Build history of the part. All positions in model axes, mm. Face numbers are marked on the shaded views. A direction names the side the tool comes from. Round coordinates to 2 decimals unless told otherwise and drop trailing zeros. Order: outer loops, then holes, each group sorted by start corner. A loop starts at its lowest first (then second) coordinate and runs counter-clockwise, first axis right, second up. Notation, with made-up numbers: (-38, -7.75) -> (-24, -7.75) arc R6 ccw to (-24, -0.75) -> close; hole circle Ø3 at (73.25, -21.75). An arc over 180 degrees is marked (long way). Use a Markdown table: item, result. Add a question column.
Item 1: Two-plate mould, pull along Z, no slides. Class the marked faces 6, 7 and 8: released by +Z, released by -Z, zero draft, split by the parting line, or undercut.
Item 2: Slice it at D-D, the plane y = 19. Give the cut face in (x, z) (3 decimals), plus the area to 3 significant figures.
Item 3: Slice it at A-A, the plane y = 9.2. Give the cut face in (x, z) (3 decimals), plus the area to 3 significant figures.
Item 4: Pin check, flat tips, straight feed: pin 1 (10 mm diameter, centred on x = -38, y = 24, fed in from -Z); pin 2 (1.5 mm diameter, centred on y = 23.5, z = 27, fed in from +X); pin 3 (10 mm diameter, centred on x = -7, y = 26.5, fed in from +Z). Stop position of each tip, or through.
Item 5: Slice it at B-B, the plane z = 3.02. Give the cut face in (x, y).
Item 6: Slice it at C-C, the plane x = -37. Give the cut face in (y, z) (3 decimals), plus the area to 3 significant figures.
Item 7: Probe L1, parallel to Y at x = -12.75, z = 3.02; L2, parallel to Y at x = -34, z = 25 (3 decimals); L3, parallel to Z at x = -17.5, y = 14.5 (3 decimals). List the from-to ranges inside material, lowest first.
Item 8: 3-axis set-ups, long thin cutter, end or side, ignore diameter. For the marked faces 1, 2, 3, 4 and 5: which of +Z, -Z, +X, -X, +Y, -Y reach the whole face in a straight line?
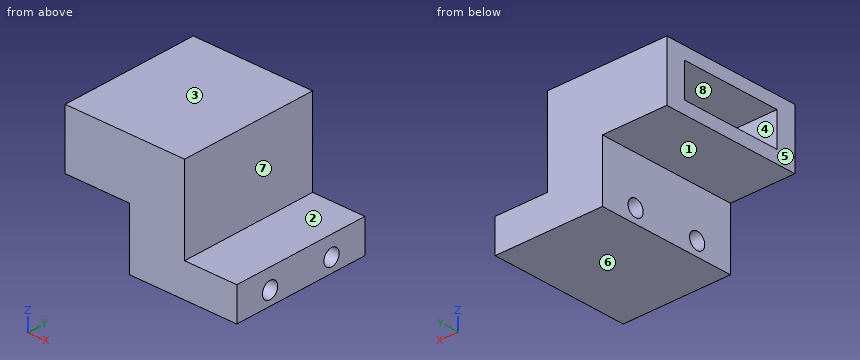
from build123d import *

# Parameters (mm, degrees)
BOSS_EXTRUDE1_DEPTH = 35.4
SKETCH2_W           = 8.63
SKETCH2_H           = 25.55
CUT_EXTRUDE1_DEPTH  = 30
SKETCH3_R           = 2.1
CUT_EXTRUDE2_DEPTH  = 64.958508207


with BuildPart() as part:
    # Sketch1 → Boss-Extrude1 (new body)
    with BuildSketch(Plane(origin=(0, 0, 0), x_dir=(1, 0, 0), z_dir=(0, 1, 0))):
        Polygon((1.0173917, 0.48), (-26.48, 0.48), (-26.48, -15), (-31.48, -15), (-43, -15), (-43, -30), (-12.38, -30), (-12.38, -8.02), (-11.48, -8.02), (1.0173917, -8.02), align=None)
    extrude(amount=BOSS_EXTRUDE1_DEPTH)

    # Sketch2 → Cut-Extrude1 (cut)
    with BuildSketch(Plane.ZY.offset(43)):
        with Locations((22.5, 17.7)):
            Rectangle(SKETCH2_W, SKETCH2_H)
    extrude(amount=-CUT_EXTRUDE1_DEPTH, mode=Mode.SUBTRACT)

    # Sketch3 → Cut-Extrude2 (cut, through all)
    with BuildSketch(Plane(origin=(1.0173917, 0, 0), x_dir=(0, 0, -1), z_dir=(1, 0, 0))):
        with Locations((-3.02, 9.2)):
            Circle(SKETCH3_R)
        with Locations((-3.02, 26.2)):
            Circle(SKETCH3_R)
    extrude(amount=-CUT_EXTRUDE2_DEPTH, mode=Mode.SUBTRACT)


solid = part.part
Check sheet entries:
| question | item | result |
|---|---|---|
| 1 | face 6 | released by -Z |
| 1 | face 7 | zero draft |
| 1 | face 8 | undercut |
| 2 | outline | (-43, 15) -> (-26.48, 15) -> (-26.48, -0.48) -> (1.017, -0.48) -> (1.017, 8.02) -> (-12.38, 8.02) -> (-12.38, 30) -> (-43, 30) -> (-43, 26.815) -> (-13, 26.815) -> (-13, 18.185) -> (-43, 18.185) -> close |
| 2 | area | 533 mm2 |
| 3 | outline | (-43, 15) -> (-26.48, 15) -> (-26.48, 5.12) -> (1.017, 5.12) -> (1.017, 8.02) -> (-12.38, 8.02) -> (-12.38, 30) -> (-43, 30) -> (-43, 26.815) -> (-13, 26.815) -> (-13, 18.185) -> (-43, 18.185) -> close; (-26.48, -0.48) -> (1.017, -0.48) -> (1.017, 0.92) -> (-26.48, 0.92) -> close |
| 3 | area | 417 mm2 |
| 4 | pin 1 | z = 15 |
| 4 | pin 2 | x = -12.38 |
| 4 | pin 3 | z = 8.02 |
| 5 | outline | (-26.48, 0) -> (1.02, 0) -> (1.02, 7.1) -> (-26.48, 7.1) -> close; (-26.48, 11.3) -> (1.02, 11.3) -> (1.02, 24.1) -> (-26.48, 24.1) -> close; (-26.48, 28.3) -> (1.02, 28.3) -> (1.02, 35.4) -> (-26.48, 35.4) -> close |
| 6 | outline | (0, 15) -> (35.4, 15) -> (35.4, 30) -> (0, 30) -> close; hole (4.925, 18.185) -> (30.475, 18.185) -> (30.475, 26.815) -> (4.925, 26.815) -> close |
| 6 | area | 311 mm2 |
| 7 | L1 | 0 to 7.1, 11.3 to 24.1, 28.3 to 35.4 |
| 7 | L2 | 0 to 4.925, 30.475 to 35.4 |
| 7 | L3 | -0.48 to 18.185, 26.815 to 30 |
| 8 | face 1 | -Z, -X, +Y, -Y |
| 8 | face 2 | +Z, +X, +Y, -Y |
| 8 | face 3 | +Z, +X, -X, +Y, -Y |
| 8 | face 4 | -X |
| 8 | face 5 | +Z, -Z, -X, +Y, -Y |
